from build123d import *

# Parameters (mm, degrees)
F0_R     = 228.6
F1_DEPTH = 6.35
F2_R     = 2.5146
F3_DEPTH = 6.35
F5_DEPTH = 6.35


with BuildPart() as f1:
    # F0 (on Top) → F1 (new body)
    with BuildSketch(Plane.XY):
        Circle(F0_R)
    extrude(amount=F1_DEPTH)

    # F2 (on face) → F3 (cut, through all)
    with BuildSketch(Plane.XY.offset(6.35)):
        with Locations((0, 48.7172)):
            Circle(F2_R)
        with Locations((28.3972, -48.744956)):
            Circle(F2_R)
        with Locations((-28.3972, -48.744956)):
            Circle(F2_R)
    extrude(amount=-F3_DEPTH, mode=Mode.SUBTRACT)

    # F4 (on face) → F5 (cut, through all)
    with BuildSketch(Plane.XY.offset(6.35)):
        with BuildLine():
            Line((157.075703, 0), (42.606701, 0))
            ThreePointArc((42.606701, 0), (34.459901, 25.056859), (13.134991, 40.531506))
            ThreePointArc((13.134991, 40.531506), (0, 63.5), (-13.134991, 40.531506))
            ThreePointArc((-13.134991, 40.531506), (-42.352335, 4.648728), (-21.614071, -36.717338))
            Line((-21.614071, -36.717338), (-21.614071, -70.620485))
            Line((-21.614071, -70.620485), (20.651158, -70.620485))
            Line((20.651158, -70.620485), (20.651158, -48.744956))
            ThreePointArc((20.651158, -48.744956), (28.382287, -40.998928), (36.143185, -48.715129))
            ThreePointArc((36.143185, -48.715129), (36.143242, -48.744956), (36.143185, -48.774783))
            Line((36.143185, -48.774783), (36.143185, -79.606533))
            Line((36.143185, -79.606533), (157.075703, -79.606533))
            Line((157.075703, -79.606533), (157.075703, 0))
        make_face()
    extrude(amount=-F5_DEPTH, mode=Mode.SUBTRACT)


solid = f1.part
Input: part model. Units: mm. Frame: model coordinates. Round coordinates to 2 decimals unless told otherwise and drop trailing zeros. Write each loop counter-clockwise with the first axis right and the second up, starting at its lowest first coordinate (ties: lowest second). Pieces come first, ordered by that corner, then holes.
1) Contact query for flat-ended pins moving along their axis: P1, Ø1.9, axis at y = -68.5, z = 3, coming from the +X side; P2, Ø1.9, axis at x = 67.5, z = 3, coming from the +Y side; P3, Ø1.9, axis at y = -60, z = 3, coming from the -X side. Output: stop coordinate, or through.
2) Ray query, L1, parallel to Y at x = 0, z = 2; L2, parallel to Y at x = 152, z = 2.75; L3, parallel to X at y = 10, z = 1.5. Return the intervals inside material, ascending.
3) Cut plane B-B (z = 3.75). Count the separate pieces of the cut face and the enclosed holes in it, then the cut area to 3 significant figures.
4) Draft query along X for faces 1 (the flat face through (48, 3, 0)), 2 (the cylindrical face through (-228.38, 10.05, 3.13)), 3 (the cylindrical face through (-42.27, 5.33, 3.22)), 4 (the cylindrical face through (34.68, 24.75, 3.22)). Return one class per face: pulls with the +X half, pulls with the -X half, needs draft (parallel to the pull), parting line crosses it, or undercut.
5) Cut plane D-D (y = 161.5). Return the cut outline in (x, z).
6) Cut plane A-A (x = 0). Return the cut outline in (y, z).
7) Cut plane C-C (y = 48.26). Return the cut outline in (x, z).
Geometry says:
1. P1: stops at x = 218.39
1. P2: stops at y = 218.7
1. P3: stops at x = -220.84
2. L1: y = -228.6 to -70.62, 63.5 to 228.6
2. L2: y = -170.75 to -79.61, 0 to 170.75
2. L3: x = -228.38 to -41.42, 41.42 to 228.38
3. separate pieces: 1
3. enclosed holes: 3
3. area: 147,000 mm2
4. face 1: needs draft
4. face 2: parting line crosses it
4. face 3: undercut
4. face 4: undercut
5. outline: (-161.79, 0) - (161.79, 0) - (161.79, 6.35) - (-161.79, 6.35) - close
6. outline: (-228.6, 0) - (-70.62, 0) - (-70.62, 6.35) - (-228.6, 6.35) - close; (63.5, 0) - (228.6, 0) - (228.6, 6.35) - (63.5, 6.35) - close
7. outline: (-223.45, 0) - (-15.24, 0) - (-15.24, 6.35) - (-223.45, 6.35) - close; (15.24, 0) - (223.45, 0) - (223.45, 6.35) - (15.24, 6.35) - close
